Input: part model. Units: mm. Frame: model coordinates. Give positions to 0.01 mm unless a question says otherwise; leave off trailing zeros. Order: outer loops, then holes, each group sorted by start corner. A loop starts at its lowest first (then second) coordinate and runs counter-clockwise, first axis right, second up. Notation, with made-up numbers: (-10.75, 70) - (40.25, 70) arc R26 cw to (40.25, 96) - close; hole circle Ø5 at (42, 40.25). An arc over 180 degrees is marked (long way). Use a Markdown table: item, result.
from build123d import *

# Parameters (mm, degrees)
SKETCH_1_W      = 32
SKETCH_1_H      = 10
SKETCH_1_R      = 3
SKETCH_1_R_2    = 2
EXTRUDE_1_DEPTH = 3
FILLET_1_R      = 5


with BuildPart() as part:
    # 草图1 → 凸台-拉伸1 (new body)
    with BuildSketch(Plane.XY):
        with Locations((9, 0)):
            Rectangle(SKETCH_1_W, SKETCH_1_H)
        Circle(SKETCH_1_R, mode=Mode.SUBTRACT)
        with Locations((20, 0)):
            Circle(SKETCH_1_R_2, mode=Mode.SUBTRACT)
    extrude(amount=EXTRUDE_1_DEPTH)

    # 圆角1
    fillet_1_edges = [part.edges().sort_by_distance(p)[0] for p in [
        (25, -5, 1.5),
        (25, 5, 1.5),
        (-7, -5, 1.5),
        (-7, 5, 1.5),
    ]]
    fillet(fillet_1_edges, radius=FILLET_1_R - 0.0001)  # a hair under: the kernel refuses the full size


solid = part.part
1. Section query A-A (x = 0). Return loops of the section in (y, z).
Response:
| item | result |
|---|---|
| outline | (-5, 0) - (-3, 0) - (-3, 3) - (-5, 3) - close; (3, 0) - (5, 0) - (5, 3) - (3, 3) - close |
2. Section query D-D (x = 19.5). Return loops of the section in (y, z).
Response:
| item | result |
|---|---|
| outline | (-5, 0) - (-1.94, 0) - (-1.94, 3) - (-5, 3) - close; (1.94, 0) - (5, 0) - (5, 3) - (1.94, 3) - close |
3. Section query C-C (y = 0.5). Return loops of the section in (x, z).
Response:
| item | result |
|---|---|
| outline | (-6.97, 0) - (-2.96, 0) - (-2.96, 3) - (-6.97, 3) - close; (2.96, 0) - (18.06, 0) - (18.06, 3) - (2.96, 3) - close; (21.94, 0) - (24.97, 0) - (24.97, 3) - (21.94, 3) - close |
4. Section query B-B (z = 2.35). State how many separate pieces and enclosed holes the cut face has, then the cut area to 3 significant figures.
Response:
| item | result |
|---|---|
| separate pieces | 1 |
| enclosed holes | 2 |
| area | 258 mm^2 |
5. Material intervals for line 1 along X through (y, z) = (1.25, 2.55); line 2 along Y through (x, z) = (20, 0.9); line 3 along X through (y, z) = (-1.75, 2.7), sorted ascending.
Response:
| item | result |
|---|---|
| line 1 | x = -6.84 to -2.73, 2.73 to 18.44, 21.56 to 24.84 |
| line 2 | y = -5 to -2, 2 to 5 |
| line 3 | x = -6.68 to -2.44, 2.44 to 19.03, 20.97 to 24.68 |
6. Mould query, pull axis Y, two halves, no side actions, for faces 1 (the face through (18.4, -1.2, 1.5)), 2 (the face through (9, 5, 1)), 3 (the face through (9, -5, 1)). Classes: pulls with the +Y half, pulls with the -Y half, needs draft (parallel to the pull), parting line crosses it, or undercut.
Response:
| item | result |
|---|---|
| face 1 | undercut |
| face 2 | pulls with the +Y half |
| face 3 | pulls with the -Y half |
